Work out the finished part from the listing and answer in its coordinate system (mm). A direction names the side the tool comes from. Give positions to 0.01 mm unless a question says otherwise; leave off trailing zeros. Order: outer loops, then holes, each group sorted by start corner. A loop starts at its lowest first (then second) coordinate and runs counter-clockwise, first axis right, second up. Notation, with made-up numbers: (8.5, 60) - (25.5, 60) arc R21 ccw to (25.5, 98) - close; hole circle Ø7 at (47, 71). An arc over 180 degrees is marked (long way). Put each result on its own line as item: value.
```python
from build123d import *

# Parameters (mm, degrees)
F0_R      = 25
F1_DEPTH  = 43
F3_DEPTH  = 25.001
F5_DEPTH  = 25.001
F7_DEPTH  = 25.001
F9_DEPTH  = 25.001
F11_DEPTH = 25.001


with BuildPart() as f1:
    # F0 (on Top) → F1 (new body)
    with BuildSketch(Plane.XY):
        Circle(F0_R)
    extrude(amount=F1_DEPTH)

    # F2 (on Front) → F3 (cut, through all)
    with BuildSketch(Plane.XZ):
        Polygon((-25.126258, 46.368178), (-13.729673, 10.771434), (-6.131949, 46.368178), align=None)
    extrude(amount=-F3_DEPTH, mode=Mode.SUBTRACT)

    # F4 (on Right) → F5 (cut, through all)
    with BuildSketch(Plane.YZ):
        Polygon((-18.553859, 10.558189), (-9.720897, 43.07955), (-24.877457, 43.07955), align=None)
        Polygon((-8.875068, 43.07955), (0, 10.558189), (6.971865, 43.07955), align=None)
    extrude(amount=-F5_DEPTH, mode=Mode.SUBTRACT)

    # F6 (on Front) → F7 (cut, through all)
    with BuildSketch(Plane.XZ):
        Polygon((15.750895, 43.012153), (-2.902546, 43.012153), (5.133678, 10.685987), align=None)
    extrude(amount=-F7_DEPTH, mode=Mode.SUBTRACT)

    # F8 (on Right) → F9 (cut, through all)
    with BuildSketch(Plane.YZ):
        Polygon((-15.306979, 10.250338), (-10.540752, 43.066985), (-24.638727, 43.066985), align=None)
        Polygon((-10.504041, 43.066985), (-10.452851, 43.066985), (-10.504041, 43.319747), (-10.540752, 43.066985), align=None)
        Polygon((-3.806771, 10.250338), (4.882272, 43.066985), (-10.452851, 43.066985), align=None)
        Polygon((4.928349, 43.066985), (4.957838, 43.066985), (4.928349, 43.241009), (4.882272, 43.066985), align=None)
        Polygon((10.518654, 10.250338), (19.207697, 43.066985), (4.957838, 43.066985), align=None)
    extrude(amount=-F9_DEPTH, mode=Mode.SUBTRACT)

    # F10 (on Right) → F11 (cut, through all)
    with BuildSketch(Plane.YZ):
        Polygon((11.531889, 10.734837), (21.7263, 43.37864), (6.711997, 43.37864), align=None)
    extrude(amount=-F11_DEPTH, mode=Mode.SUBTRACT)


solid = f1.part
```
(1) Determine the mould class of faces 1 (the face through (-15.172, 16.152, 15.277)), 2 (the face through (10.366, 12.062, 26.617)), 3 (the face through (0, 0, 0)), 4 (the face through (0, -7, 30)) for opening direction X: pulls with the +X half, pulls with the -X half, needs draft (parallel to the pull), parting line crosses it, or undercut.
Geometry check:
face 1: undercut
face 2: undercut
face 3: needs draft
face 4: pulls with the -X half
(2) Section D-D, the plane y = -22 is taken. Write down the section's boundary in (x, z), then the cut area to 3 significant figures.
Geometry check:
outline: (-11.87, 0) - (11.87, 0) - (11.87, 43) - (0, 43) - (0, 28.28) - (-11.87, 28.28) - close
area: 846 mm²
(3) Section C-C, the plane x = -5 is taken. Write down the section's boundary in (y, z).
Geometry check:
outline: (-24.49, 0) - (24.49, 0) - (24.49, 43) - (21.61, 43) - (11.53, 10.73) - (11.22, 12.88) - (10.52, 10.25) - (5.85, 37.83) - (0, 10.56) - (-1.89, 17.49) - (-3.81, 10.25) - (-10.14, 41.53) - (-11.48, 36.61) - (-15.31, 10.25) - (-17.01, 16.24) - (-18.55, 10.56) - (-24.49, 41.11) - close
(4) A tool of negligible diameter and unlimited length cuts with its end or side. For faces 5 (the face through (14, -7, 43)), 6 (the face through (-12.166, 5.165, 18.097)), 7 (the face through (-11.27, -10.82, 39.03)), from which of +Z, -Z, +X, -X, +Y, -Y can it reach the whole face along a straight path? Write none if from no direction.
Geometry check:
face 5: +Z, +X, -X, +Y, -Y
face 6: +Z, +Y
face 7: +Z, -X
(5) Section A-A, the plane z = 35.5 is taken. Write down the section's boundary in (x, y) (1 decimal).
Geometry check:
outline: (-24.4, 5.3) - (-21.6, 5.3) - (-21.6, 6.2) - (-24.2, 6.2) arc R25 ccw to start; (-23.4, -8.9) arc R25 ccw to (-22.1, -11.6) - (0, -11.6) - (0, -23.4) - (-8.8, -23.4) arc R25 ccw to (13.3, 21.2) - (13.3, 0) - (0, 0) - (0, -8.9) - close; (-8.5, 5.3) - (-1, 5.3) - (-1, 6.2) - (-8.5, 6.2) - close; (-8.5, 19.3) - (-1, 19.3) - (-1, 25) arc R25 ccw to (-8.5, 23.5) - close
(6) Section B-B, the plane z = 22 is taken. Write down the section's boundary in (x, y).
Geometry check:
outline: (-24.88, 2.45) - (-17.32, 2.45) - (-17.32, 8.53) - (-23.5, 8.53) arc R25 ccw to start; (-24.22, -6.19) arc R25 ccw to (-20.98, -13.6) - (0, -13.6) - (0, -20.78) - (-13.9, -20.78) arc R25 ccw (long way) to (8.85, 23.38) - (8.85, 0) - (2.32, 0) - (2.32, 24.89) arc R25 ccw to (-11.33, 22.28) - (-11.33, 15.05) - (0, 15.05) - (0, 8.53) - (-11.33, 8.53) - (-11.33, 2.45) - (0, 2.45) - (0, -6.19) - close; (-19.96, 15.05) - (-17.32, 15.05) - (-17.32, 18.02) arc R25 ccw to start
(7) Straight lines are drawn through the part: line 1 (Y direction, x = -18.5, z = 20.5); line 2 (Y direction, x = -4.5, z = 37); line 3 (X direction, y = 14.5, z = 30). For each, find the intervals that lie inside material, in ascending order.
Geometry check:
line 1: y = -13.82 to -5.88, 2.13 to 8.78, 14.58 to 16.82
line 2: y = -24.59 to -23.7, -11.37 to -9.22, 5.67 to 5.99, 19.73 to 24.59
line 3: x = 0 to 0.33, 11.48 to 20.37
(8) Given pin 1 (5 mm diameter, centred on x = 7, y = 15, fed in from -Z); pin 2 (5.5 mm diameter, centred on y = 11.5, z = 23, fed in from -X); pin 3 (12 mm diameter, centred on x = -19.5, z = 25.5, fed in from -Y); pin 4 (4.5 mm diameter, centred on x = 7.5, z = 24.5, fed in from +Y), each flat-ended and moving along its own axis, determine where each tip first touches the part or whether it passes through.
Geometry check:
pin 1: stops at z = 0
pin 2: stops at x = 0
pin 3: stops at y = -13.96
pin 4: stops at y = 23.25
